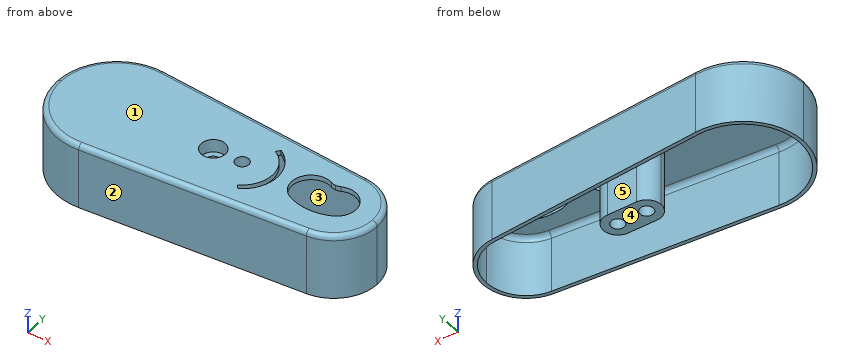
from build123d import *
from build123d.topology import SkipClean

# Parameters (mm, degrees)
AUFSATZ_LINEAR_AUSTRAGEN1_DEPTH                      = 25
AUFSATZ_LINEAR_AUSTRAGEN2_DEPTH                      = 2
VERRUNDUNG1_R                                        = 2
SCHNITT_LINEAR_AUSTRAGEN1_REACH                      = 116.096
AUFSATZ_LINEAR_AUSTRAGEN3_DEPTH                      = 25
SPIEGELN2_DEPTH                                      = 25
STIRNSENKUNG_F_R_M5_ZYLINDERSCHRAUBE_MIT_D           = 5.5
STIRNSENKUNG_F_R_M5_ZYLINDERSCHRAUBE_MIT_CBORE_D     = 10
STIRNSENKUNG_F_R_M5_ZYLINDERSCHRAUBE_MIT_CBORE_DEPTH = 5.4
DURCHGANGSLOCH_F_R_M51_D                             = 5.5
SCHNITT_LINEAR_AUSTRAGEN2_REACH                      = 116.096


# Read off the part's stored shape, not the designer's step: Spiegeln2
with BuildPart() as part:
    # Skizze1 → Aufsatz-Linear austragen1 (new body)
    with BuildSketch(Plane.XY):
        with BuildLine():
            Line((1.944444444, 24.924268009), (91.4, 17.945472967))
            ThreePointArc((91.4, 17.945472967), (103.213629327, 12.222929272), (108, 0))
            Line((108, 0), (106.5, 0))
            ThreePointArc((106.5, 0), (102.11249355, 11.204351833), (91.283333333, 16.450016886))
            Line((91.283333333, 16.450016886), (1.827777778, 23.428811929))
            ThreePointArc((1.827777778, 23.428811929), (-15.957713217, 17.251127177), (-23.5, 0))
            Line((-23.5, 0), (-25, 0))
            ThreePointArc((-25, 0), (-16.976290656, 18.352262955), (1.944444444, 24.924268009))
        make_face()
    extrude(amount=AUFSATZ_LINEAR_AUSTRAGEN1_DEPTH)

    # Skizze2 → Aufsatz-Linear austragen2 (add)
    with BuildSketch(Plane.XY.offset(25)):
        with BuildLine():
            Line((108, 0), (-25, 0))
            ThreePointArc((-25, 0), (-16.976290656, 18.352262955), (1.944444444, 24.924268009))
            Line((1.944444444, 24.924268009), (91.4, 17.945472967))
            ThreePointArc((91.4, 17.945472967), (103.213629327, 12.222929272), (108, 0))
        make_face()
    extrude(amount=AUFSATZ_LINEAR_AUSTRAGEN2_DEPTH)

    # Verrundung1
    verrundung1_edges = [part.edges().sort_by_distance(p)[0] for p in [
        (-15.957713217, 17.251127177, 25),
        (46.555555556, 19.939414407, 25),
        (-16.976290656, 18.352262955, 27),
        (102.11249355, 11.204351833, 25),
        (103.213629327, 12.222929272, 27),
        (46.672222222, 21.434870488, 27),
    ]]
    fillet(verrundung1_edges, radius=VERRUNDUNG1_R)

    # Spiegeln1: part across plane


with BuildPart() as part_1:
    with SkipClean():  # the faces are left unmerged after this step: merging them gives an invalid solid
        add(part.part)
        add(part.part.mirror(Plane.ZX))

    # Skizze11 → Schnitt-Linear austragen1 (cut, up to next)
    with BuildSketch(Plane.XY.offset(27), mode=Mode.PRIVATE) as schnitt_linear_austragen1_sk1:
        with BuildLine():
            Line((85, 0), (85, 8))
            ThreePointArc((85, 8), (85.973978263, 8.106667968), (86.901782178, 8.421614958))
            ThreePointArc((86.901782178, 8.421614958), (97.533190568, 4.552098756), (93.663674366, -6.079309634))
            ThreePointArc((93.663674366, -6.079309634), (89.437012086, -7.514068146), (85, -8))
            Line((85, -8), (85, 0))
        make_face()
    schnitt_linear_austragen1_tool1 = extrude(schnitt_linear_austragen1_sk1.sketch, amount=-SCHNITT_LINEAR_AUSTRAGEN1_REACH, mode=Mode.PRIVATE) & part_1.part
    schnitt_linear_austragen1 = schnitt_linear_austragen1_tool1.solids().sort_by_distance((90.892741, 0.809501, 27))[0]
    add(schnitt_linear_austragen1, mode=Mode.SUBTRACT)

    # Spiegeln3: Schnitt-Linear austragen1 across plane
    with SkipClean():  # the faces are left unmerged after this step: merging them gives an invalid solid
        add(schnitt_linear_austragen1.mirror(Plane(origin=(85, 0, -0.001), x_dir=(0, 0, 1), z_dir=(-1, 0, 0))), mode=Mode.SUBTRACT)

    # Skizze3 → Aufsatz-Linear austragen3 (add)
    with SkipClean():  # the faces are left unmerged after this step: merging them gives an invalid solid
        with BuildSketch(Plane.XY):
            with BuildLine():
                Line((46, 6), (46, 0))
                Line((46, 0), (34, 0))
                ThreePointArc((34, 0), (35.757359313, 4.242640687), (40, 6))
                Line((40, 6), (46, 6))
            make_face()
        extrude(amount=AUFSATZ_LINEAR_AUSTRAGEN3_DEPTH)

    # Spiegeln2 outline → Spiegeln2 (add)
    with SkipClean():  # the faces are left unmerged after this step: merging them gives an invalid solid
        with BuildSketch(Plane.XY):
            with BuildLine():
                Line((52, 6), (46, 6))
                Line((46, 6), (46, 0))
                Line((46, 0), (34, 0))
                ThreePointArc((34, 0), (35.757359313, -4.242640687), (40, -6))
                Line((40, -6), (52, -6))
                ThreePointArc((52, -6), (58, 0), (52, 6))
            make_face()
        extrude(amount=SPIEGELN2_DEPTH)

    # Stirnsenkung für M5 Zylinderschraube mit Innensechskant2 (through all)
    with Locations(Plane.XY.offset(27)):
        with Locations((40, 0)):
            CounterBoreHole(STIRNSENKUNG_F_R_M5_ZYLINDERSCHRAUBE_MIT_D / 2, STIRNSENKUNG_F_R_M5_ZYLINDERSCHRAUBE_MIT_CBORE_D / 2, STIRNSENKUNG_F_R_M5_ZYLINDERSCHRAUBE_MIT_CBORE_DEPTH)

    # Durchgangsloch für M51 (through all)
    with Locations(Plane.XY.offset(27)):
        with Locations((52, 0)):
            Hole(DURCHGANGSLOCH_F_R_M51_D / 2)

    # Skizze12 → Schnitt-Linear austragen2 (cut, up to next)
    with BuildSketch(Plane.XY.offset(27), mode=Mode.PRIVATE) as schnitt_linear_austragen2_sk1:
        with BuildLine():
            Line((59.155963734, -12.611192768), (57.924777873, -11.006680115))
            ThreePointArc((57.924777873, -11.006680115), (64.5, 0), (57.924777873, 11.006680115))
            Line((57.924777873, 11.006680115), (59.155963734, 12.611192768))
            ThreePointArc((59.155963734, 12.611192768), (60.01066697, 12.086323457), (60.827040721, 11.503623434))
            ThreePointArc((60.827040721, 11.503623434), (66.5, 0), (60.827040721, -11.503623434))
            ThreePointArc((60.827040721, -11.503623434), (60.01066697, -12.086323457), (59.155963734, -12.611192768))
        make_face()
    schnitt_linear_austragen2_tool1 = extrude(schnitt_linear_austragen2_sk1.sketch, amount=-SCHNITT_LINEAR_AUSTRAGEN2_REACH, mode=Mode.PRIVATE) & part_1.part
    add(schnitt_linear_austragen2_tool1.solids().sort_by_distance((58.751722, -11.646761, 27))[0], mode=Mode.SUBTRACT)


solid = part_1.part
Could you check a few things on this model? Use its own coordinates, in mm. Face numbers are marked on the shaded views. A direction names the side the tool comes from. Give positions to 0.01 mm unless a question says otherwise; leave off trailing zeros. Write each loop counter-clockwise with the first axis right and the second up, starting at its lowest first coordinate (ties: lowest second). Pieces come first, ordered by that corner, then holes. Notation, with made-up numbers: (84, 44) -> (132, 44) arc R12 cw to (132, 62) -> close; hole circle Ø7 at (29.25, 73.5). An arc over 180 degrees is marked (long way). Answer as a JSON object with one key per item and string values.
Q1. Please list where these lines run through material, in increasing order: L1, parallel to Y at x = 40, z = 7.25; L2, parallel to X at y = 1, z = 20; L3, parallel to X at y = 4, z = 9.5.
Taken from the geometry:
{"L1": "y = -21.96 to -20.45, -6 to -2.75, 2.75 to 6, 20.45 to 21.96", "L2": "x = -24.98 to -23.48, 34.08 to 37.44, 42.56 to 49.44, 54.56 to 57.92, 106.47 to 107.97", "L3": "x = -24.68 to -23.16, 35.53 to 56.47, 106.01 to 107.55"}
Q2. Suppose I cut it at A-A on z = 2.5. Write out the boundary of the cut face in (x, y), then the cut area to 3 significant figures.
Taken from the geometry:
{"outline": "(1.94, -24.92) -> (91.4, -17.95) arc R18 ccw to (91.4, 17.95) -> (1.94, 24.92) arc R25 ccw (long way) to start; (40, -6) -> (52, -6) arc R6 ccw to (52, 6) -> (40, 6) arc R6 ccw to start; hole (1.83, -23.43) -> (91.28, -16.45) arc R16.5 ccw to (91.28, 16.45) -> (1.83, 23.43) arc R23.5 ccw (long way) to start; hole circle Ø5.5 at (40, 0); hole circle Ø5.5 at (52, 0)", "area": "676 mm²"}
Q3. We'd pull the mould along X, two halves only. Please class the marked faces 1, 2 and 3: released by +X, released by -X, zero draft, split by the parting line, or undercut.
Taken from the geometry:
{"face 1": "zero draft", "face 2": "released by +X", "face 3": "undercut"}
Q4. Which directions (+Z, -Z, +X, -X, +Y, -Y) give clear straight access to the entire face, cutting with the end or side of a thin tool? Please do the marked faces 4 and 5.
Taken from the geometry:
{"face 4": "-Z, +X, -X, +Y, -Y", "face 5": "-Z"}
Q5. Will these pins go through, and if not, where does the flat tip stop? pin 1 Ø13 at (x, y) = (18.5, 9) entering from -Z; pin 2 Ø3 at (x, y) = (40, -1) entering from +Z; pin 3 Ø12 at (x, y) = (-8.5, 15) entering from -Z; pin 4 Ø6 at (x, z) = (48, 18) entering from +Y.
Taken from the geometry:
{"pin 1": "stops at z = 25", "pin 2": "passes through", "pin 3": "stops at z = 23.98", "pin 4": "stops at y = 21.57"}
